Read the model definition and answer for the solid it produces. Units are mm, in the model's axes. Round coordinates to 2 decimals unless told otherwise and drop trailing zeros. Write each loop counter-clockwise with the first axis right and the second up, starting at its lowest first coordinate (ties: lowest second). Pieces come first, ordered by that corner, then holes. Notation, with made-up numbers: (48, -17) -> (91, -17) arc R30 cw to (91, 21) -> close; hole circle Ø10 at (7.25, 79). An arc over 180 degrees is marked (long way). Return JSON: item names as keys, results as strings.
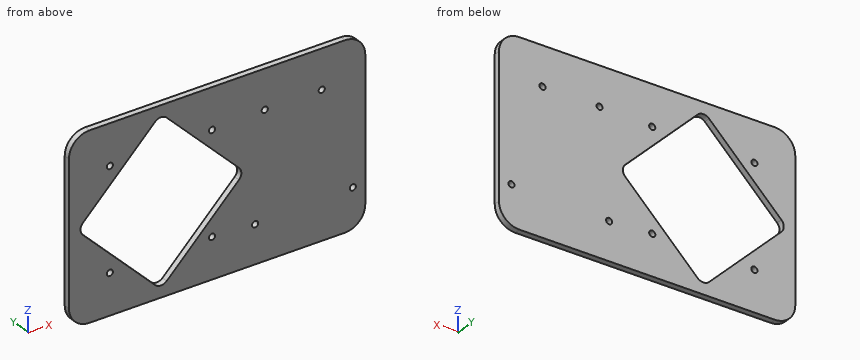
from build123d import *

# Parameters (mm, degrees)
BASE_W                     = 145
BASE_H                     = 90
RESSALTO_EXTRUS_O1_DEPTH   = 3
CORTE_EXTRUS_O1_DEPTH      = 86.382960829
FURO_DE_DI_METRO_3_0_3_1_D = 3
FURO_DE_DI_METRO_3_0_3_7_D = 3
FILETE1_R                  = 10
FILETE2_R                  = 4


with BuildPart() as part:
    # Base → Ressalto-extrusão1 (new body)
    with BuildSketch(Plane(origin=(0, 0, 0), x_dir=(1, 0, 0), z_dir=(0, 1, 0))):
        Rectangle(BASE_W, BASE_H)
    extrude(amount=-RESSALTO_EXTRUS_O1_DEPTH)

    # Recorte → Corte-extrusão1 (cut, through all)
    with BuildSketch(Plane(origin=(0, 0, 0), x_dir=(1, 0, 0), z_dir=(0, 1, 0))):
        Polygon((-68.512193309, 0), (-27.5, 41.012193309), (13.512193309, 0), (-27.5, -41.012193309), align=None)
    extrude(amount=-CORTE_EXTRUS_O1_DEPTH, mode=Mode.SUBTRACT)

    # Furo de diâmetro Ø3.0 (3)1 (through all)
    with Locations(Plane(origin=(0, 0, 0), x_dir=(1, 0, 0), z_dir=(0, 1, 0))):
        with Locations((-52.5, 25), (-2.5, 25), (-2.5, -25), (-52.5, -25)):
            Hole(FURO_DE_DI_METRO_3_0_3_1_D / 2)

    # Furo de diâmetro Ø3.0 (3)7 (through all)
    with Locations(Plane(origin=(0, 0, 0), x_dir=(1, 0, 0), z_dir=(0, 1, 0))):
        with Locations((18.6, 26.225), (23.3, -25.675), (51.2, -25.675), (66.4, 25.125)):
            Hole(FURO_DE_DI_METRO_3_0_3_7_D / 2)

    # Filete1
    filete1_edges = [part.edges().sort_by_distance(p)[0] for p in [
        (72.5, -1.5, 45),
        (-72.5, -1.5, 45),
        (-72.5, -1.5, -45),
        (72.5, -1.5, -45),
    ]]
    fillet(filete1_edges, radius=FILETE1_R)

    # Filete2
    filete2_edges = [part.edges().sort_by_distance(p)[0] for p in [
        (-68.512193309, -1.5, 0),
        (-27.5, -1.5, -41.012193309),
        (13.512193309, -1.5, 0),
        (-27.5, -1.5, 41.012193309),
    ]]
    fillet(filete2_edges, radius=FILETE2_R)


solid = part.part
Item 1: Section A-A (x = 51.2) is taken. Give the vertices of the cut face in (y, z) (3 decimals), then the cut area to 3 significant figures.
Worked answers:
{"outline": "(-3, -45) -> (0, -45) -> (0, 24.175) -> (-3, 24.175) -> close; (-3, 27.175) -> (0, 27.175) -> (0, 45) -> (-3, 45) -> close", "area": "261 mm2"}
Item 2: Section B-B (z = 1) is taken. Give the vertices of the cut face in (x, y), then the cut area to 3 significant figures.
Worked answers:
{"outline": "(-72.5, -3) -> (-66.73, -3) -> (-66.73, 0) -> (-72.5, 0) -> close; (11.73, -3) -> (72.5, -3) -> (72.5, 0) -> (11.73, 0) -> close", "area": "200 mm2"}
Item 3: Straight lines are drawn through the part: L1, parallel to X at y = -2.3, z = 25; L2, parallel to X at y = -1.9, z = -25; L3, parallel to Z at x = 23.3, y = -1.95 (3 decimals). For each, find the intervals that lie inside material, in ascending order. Write a range as [from, to].
Worked answers:
{"L1": "x = [-72.5, -54], [-51, -43.51], [-11.49, -4], [-1, 21.96], [24.64, 49.86], [52.54, 72.5]", "L2": "x = [-72.5, -54], [-51, -43.51], [-11.49, -4], [-1, 17.73], [19.47, 64.91], [67.89, 72.5]", "L3": "z = [-45, 24.175], [27.175, 45]"}
Item 4: Section C-C (y = -1) is taken. State how many separate pieces and enclosed holes the cut face has, then the cut area to 3 significant figures.
Worked answers:
{"separate pieces": "1", "enclosed holes": "9", "area": "9,560 mm2"}
Item 5: A flat-ended cylindrical pin translates along its axis: pin 1 (2.5 mm diameter, centred on x = 51.2, z = 25.675, fed in from +Y). Find the tip coordinate at first contact, or state that the pin passes through.
Worked answers:
{"pin 1": "passes through"}
